from build123d import *

# Parameters (mm, degrees)
RESSALTO_EXTRUS_O1_DEPTH = 10
ESBO_O2_R                = 2
CORTE_EXTRUS_O1_DEPTH    = 20
ESBO_O4_W                = 7
ESBO_O4_H                = 10
CORTE_EXTRUS_O2_DEPTH    = 20


with BuildPart() as part:
    # Esboço1 → Ressalto-extrusão1 (new body)
    with BuildSketch(Plane.XY):
        Polygon((32, 0), (32, 15), (0, 15), (0, 0), (10, 0), (10, 10), (22, 10), (22, 0), align=None)
    extrude(amount=RESSALTO_EXTRUS_O1_DEPTH)

    # Esboço2 → Corte-extrusão1 (cut)
    with BuildSketch(Plane(origin=(0, 0, 0), x_dir=(-1, 0, 0), z_dir=(0, -1, 0))):
        with Locations((-4, -5)):
            Circle(ESBO_O2_R)
        with Locations((-28, -5)):
            Circle(ESBO_O2_R)
    extrude(amount=-CORTE_EXTRUS_O1_DEPTH, mode=Mode.SUBTRACT)

    # Esboço4 → Corte-extrusão2 (cut)
    with BuildSketch(Plane(origin=(0, 0, 0), x_dir=(-1, 0, 0), z_dir=(0, 0, -1))):
        with Locations((-28.5, 10)):
            Rectangle(ESBO_O4_W, ESBO_O4_H)
        with Locations((-3.5, 10)):
            Rectangle(ESBO_O4_W, ESBO_O4_H)
    extrude(amount=-CORTE_EXTRUS_O2_DEPTH, mode=Mode.SUBTRACT)


solid = part.part
Source: CAD feature listing. Evaluate the final solid. Frame: model axes, mm. A direction names the side the tool comes from. Coordinates: 2 decimals unless noted, no trailing zeros. Loops run counter-clockwise (first coordinate to the right, second up) from the corner with the lowest first, then second, coordinate; pieces in that order, holes last. Notation, with made-up numbers: M 71.25,64 L 113.25,64 A13 cw 113.25,79 Z; hole C -3.75,-29 d5. An arc over 180 degrees is marked long. Answer in a Markdown table with one row per item.
Q1. Section C-C on y = 9.5. Return the cut outline in (x, z), plus the area to 3 significant figures.
Answers below:
| item | result |
|---|---|
| outline | M 7,0 L 10,0 L 10,10 L 7,10 Z; M 22,0 L 25,0 L 25,10 L 22,10 Z |
| area | 60.0 mm^2 |
Q2. Ray query, probe 1 along X at (y, z) = (2.35, 5); probe 2 along X at (y, z) = (9.5, 4.5); probe 3 along Z at (x, y) = (28, 2.6). Return the intervals inside material, ascending. Write a range as from..to.
Answers below:
| item | result |
|---|---|
| probe 1 | x = 0..2, 6..10, 22..26, 30..32 |
| probe 2 | x = 7..10, 22..25 |
| probe 3 | z = 0..3, 7..10 |
Q3. Section A-A on y = 3.75. Return the cut outline in (x, z).
Answers below:
| item | result |
|---|---|
| outline | M 0,0 L 10,0 L 10,10 L 0,10 Z; M 22,0 L 32,0 L 32,10 L 22,10 Z; hole C 4,5 d4; hole C 28,5 d4 |
Q4. First-contact query: pin 1 (3 mm diameter, centred on y = 12, z = 3, fed in from -X); pin 2 (5 mm diameter, centred on x = 3.5, z = 3, fed in from +Y); pin 3 (3 mm diameter, centred on y = 9.5, z = 4.5, fed in from +X). Flat tips, straight axial feed; report the tip coordinate or a pass-through.
Answers below:
| item | result |
|---|---|
| pin 1 | stops at x = 7 |
| pin 2 | stops at y = 5 |
| pin 3 | stops at x = 25 |
Q5. Set-up query: faces 1 (the flat face through (30, 5, 4)), 2 (the flat face through (2, 5, 4)), 3 (the flat face through (16, 10, 5)). Return all of +Z, -Z, +X, -X, +Y, -Y with unobstructed straight access to the full face (end or side cutting, diameter ignored); none if empty.
Answers below:
| item | result |
|---|---|
| face 1 | +Z, -Z, +X, +Y |
| face 2 | +Z, -Z, -X, +Y |
| face 3 | +Z, -Z, -Y |
Q6. Section D-D on z = 5. Return the cut outline in (x, y).
Answers below:
| item | result |
|---|---|
| outline | M 0,0 L 2,0 L 2,5 L 0,5 Z; M 6,0 L 10,0 L 10,10 L 22,10 L 22,0 L 26,0 L 26,5 L 25,5 L 25,15 L 7,15 L 7,5 L 6,5 Z; M 30,0 L 32,0 L 32,5 L 30,5 Z |
Q7. Section B-B on x = 28. Return the cut outline in (y, z), plus the area to 3 significant figures.
Answers below:
| item | result |
|---|---|
| outline | M 0,0 L 5,0 L 5,3 L 0,3 Z; M 0,7 L 5,7 L 5,10 L 0,10 Z |
| area | 30.0 mm^2 |
